```python
from build123d import *


with BuildPart() as f3:
    # F0 (on Top) → F3 section 0
    with BuildSketch(Plane.XY, mode=Mode.PRIVATE) as f3_s0:
        Polygon((-22.561089, -40.85453), (24.100516, -39.965741), (46.661605, 0.888788), (22.561089, 40.85453), (-24.100516, 39.965741), (-46.661605, -0.888788), align=None)
    loft([f3_s0.sketch, Vertex(0, 0, 125)])


solid = f3.part
```
Here's how the part is built. I have some questions about the finished solid (model axes, mm). Give positions to 0.01 mm unless a question says otherwise; leave off trailing zeros. Write each loop counter-clockwise with the first axis right and the second up, starting at its lowest first coordinate (ties: lowest second). Pieces come first, ordered by that corner, then holes.
(1) If I drill on L1, parallel to Y at x = 8.5, z = 12; L2, parallel to X at y = 30, z = 27.5; L3, parallel to X at y = 0.5, z = 76.5, over which ranges is the centre line in solid material (lowest first)?
Output values:
L1: y = -36.38 to 36.71
L2: x = -19.45 to 18.72
L3: x = -17.64 to 18.01
(2) Imagine slicing it at C-C, the plane y = 35.5. Write out the boundary of the cut face in (x, z), and give its area (3 significant figures).
Output values:
outline: (-26.57, 0) - (25.79, 0) - (19.6, 16.38) - (-21.41, 13.97) - close
area: 709 mm2
(3) Imagine slicing it at B-B, the plane z = 100.5. Write out the boundary of the cut face in (x, y).
Output values:
outline: (-9.15, -0.17) - (-4.42, -8.01) - (4.72, -7.83) - (9.15, 0.17) - (4.42, 8.01) - (-4.72, 7.83) - close
(4) Imagine slicing it at A-A, the plane x = 17.5. Write out the boundary of the cut face in (y, z).
Output values:
outline: (-40.09, 0) - (40.76, 0) - (31.69, 28.04) - (0.33, 78.12) - (-29.02, 34.23) - close
(5) Imagine slicing it at D-D, the plane z = 36.5. Write out the boundary of the cut face in (x, y) (3 decimals).
Output values:
outline: (-33.036, -0.629) - (-15.973, -28.925) - (17.063, -28.296) - (33.036, 0.629) - (15.973, 28.925) - (-17.063, 28.296) - close
(6) Will these pins go through, and if not, where does the flat tip stop? pin 1 (8 mm diameter, centred on x = 1, z = 67, fed in from +Y); pin 2 (1 mm diameter, centred on x = -1.5, z = 91.5, fed in from +Y); pin 3 (12 mm diameter, centred on x = -33, z = 30.5, fed in from +Y).
Output values:
pin 1: stops at y = 20.07
pin 2: stops at y = 10.97
pin 3: stops at y = 15.03
